For this review, take the finished solid that the model builds, in its own axes (mm). Face numbers are marked on the shaded views. A direction names the side the tool comes from. Coordinates: 2 decimals unless noted, no trailing zeros. Write each loop counter-clockwise with the first axis right and the second up, starting at its lowest first coordinate (ties: lowest second). Pieces come first, ordered by that corner, then holes. Notation, with made-up numbers: M 24,76 L 40,76 A27 ccw 40,108 Z; hole C 81,57 d7. An arc over 180 degrees is marked long. One line per question, with ' | ' between items.
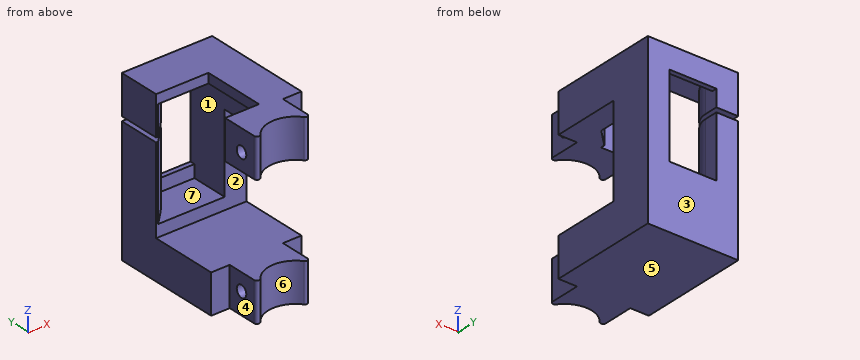
Autodesk Inventor part; units mm, degrees
ref_plane "YZ Plane" through (0, 0, 0) normal (1, 0, 0) x (0, 1, 0)
ref_plane "XZ Plane" through (0, 0, 0) normal (0, 1, 0) x (-1, 0, 0)
ref_plane "XY Plane" through (0, 0, 0) normal (0, 0, 1) x (1, 0, 0)
sketch "Side Block" plane through (0, 0, 0) normal (0, 0, 1) x (1, 0, 0)
  line L0 (11.2978, -7.5275) -> (11.2978, -16.0456)
  line L1 (11.2978, -7.5275) -> (16.5429, -7.5275)
  line L2 (16.5429, -7.5275) -> (16.5429, 23.5875)
  line L3 (16.5429, 23.5875) -> (-8.9841, 23.5875)
  line L4 (-8.9841, 23.5875) -> (-8.9841, -7.5275)
  line L5 (-8.9841, -7.5275) -> (-3.739, -7.5275)
  line L6 (-3.739, -16.0456) -> (-3.739, -7.5275)
  line L7 (3.7794, -23.2501) -> (3.7794, -21.2181)
  arc A0 (9.9308, -16.5088) -> (-2.3719, -16.5088) centre (3.7794, -21.2181) ccw
  arc A1 (-3.739, -16.0456) -> (-2.3719, -16.5088) centre (-2.977, -16.0456) ccw
  arc A2 (9.9308, -16.5088) -> (11.2978, -16.0456) centre (10.5358, -16.0456) ccw
  point P0 (3.7794, -4.0139)
  point P1 (-3.739, -19.35)
  point P2 (11.2978, -19.35)
  dimension "d2" = 31.115
  dimension "d3" = 31.115
  dimension "d4" = 5.2451
  dimension "d5" = 25.527
  dimension "d58" = 2.032
  dimension "d59" = 15.494
  dimension "d60" = 0.762
sketch "Motor Containment" plane through (0, 0, 0) normal (0, 0, 1) x (1, 0, 0)
  line L0 (-35.1538, -13.4444) -> (-35.1538, -17.0004) construction
  line L1 (-35.1538, -40.3684) -> (-35.1538, -43.9244) construction
  line L2 (-35.1538, -17.0004) -> (-35.1538, -22.8424)
  line L3 (-41.7578, -43.9244) -> (-28.5498, -43.9244)
  line L4 (-28.5498, -43.9244) -> (-28.5498, -13.4444)
  line L5 (-28.5498, -13.4444) -> (-41.7578, -13.4444)
  line L6 (-41.7578, -13.4444) -> (-41.7578, -43.9244)
  line L7 (-41.7578, -40.3684) -> (-28.5498, -40.3684)
  line L8 (-28.5498, -40.3684) -> (-28.5498, -17.0004)
  line L9 (-28.5498, -17.0004) -> (-41.7578, -17.0004)
  line L10 (-41.7578, -17.0004) -> (-41.7578, -40.3684)
  point P0 (-35.1538, -28.1145)
  dimension "d17" = 13.208
  dimension "d18" = 30.48
  dimension "d19" = 23.368
  dimension "d20" = 5.842
sketch "Sketch1" plane through (0, 0, 0) normal (0, 0, 1) x (1, 0, 0)
  line L0 (11.2978, -7.5275) -> (11.2978, -16.0456)
  line L1 (11.2978, -7.5275) -> (16.5429, -7.5275)
  line L2 (16.5429, -7.5275) -> (16.5429, 23.5875)
  line L3 (16.5429, 23.5875) -> (-8.9841, 23.5875)
  line L4 (-8.9841, 23.5875) -> (-8.9841, -7.5275)
  line L5 (-8.9841, -7.5275) -> (-3.739, -7.5275)
  line L6 (-3.739, -16.0456) -> (-3.739, -7.5275)
  line L7 (3.7794, -23.2501) -> (3.7794, -21.2181)
  arc A0 (9.9308, -16.5088) -> (-2.3719, -16.5088) centre (3.7794, -21.2181) ccw
  arc A1 (-3.739, -16.0456) -> (-2.3719, -16.5088) centre (-2.977, -16.0456) ccw
  arc A2 (9.9308, -16.5088) -> (11.2978, -16.0456) centre (10.5358, -16.0456) ccw
  point P0 (0, 0)
  dimension "d6" = 23.5875
extrude "Extrusion1" add sketch "Sketch1" along normal blind 47.5742
sketch "Sketch2" plane through (-8.9841, 23.5875, 0) normal (0, 1, 0) x (1, 0, 0)
  line L0 (0, -47.5742) -> (5.2451, -47.5742)
  line L1 (20.2819, 0) -> (25.527, 0)
  line L2 (0, -47.5742) -> (25.527, -47.5742)
  line L3 (25.527, -47.5742) -> (25.527, 0)
  line L4 (25.527, 0) -> (0, 0)
  line L5 (0, 0) -> (0, -47.5742)
  line L6 (0, -23.7871) -> (25.527, -23.7871) construction
  circle A0 centre (12.7635, -23.7871) radius 12.7
  line L7 (0, 0) -> (0, -47.5742)
  line L8 (0, -11.0871) -> (25.527, -11.0871)
  line L9 (12.7635, -14.3891) -> (12.7635, -17.9451) construction
  line L10 (12.7635, -41.3131) -> (12.7635, -44.8691) construction
  line L11 (12.7635, -17.9451) -> (12.7635, -23.7871)
  line L12 (6.1595, -44.8691) -> (19.3675, -44.8691)
  line L13 (19.3675, -44.8691) -> (19.3675, -14.3891)
  line L14 (19.3675, -14.3891) -> (6.1595, -14.3891)
  line L15 (6.1595, -14.3891) -> (6.1595, -44.8691)
  line L16 (6.1595, -41.3131) -> (19.3675, -41.3131)
  line L17 (19.3675, -41.3131) -> (19.3675, -17.9451)
  line L18 (19.3675, -17.9451) -> (6.1595, -17.9451)
  line L19 (6.1595, -17.9451) -> (6.1595, -41.3131)
  point P0 (8.9841, 0)
  point P1 (6.1595, -17.9451)
  dimension "d21" = 25.4
sketch "Sketch3" plane through (-8.9841, -7.5275, 0) normal (-1, 0, 0) x (0, 0, 1)
  line L0 (0, 19.177) -> (47.5742, 19.177)
  line L1 (47.5742, 31.115) -> (47.5742, 0)
  line L2 (0, 31.115) -> (47.5742, 31.115)
  line L3 (41.4528, 31.115) -> (41.4528, -19.3537) construction
  line L4 (6.1214, 31.115) -> (6.1214, -20.7554) construction
  line L5 (0, 31.115) -> (0, 0) construction
  circle A0 centre (6.1214, -4.1148) radius 1.6637
  circle A1 centre (41.4528, -4.1148) radius 1.6637
  line L6 (23.7871, 31.115) -> (23.7871, -19.3537) construction
  line L7 (36.576, 19.177) -> (36.576, -23.6144)
  line L8 (10.9982, 19.177) -> (10.9982, -23.6144)
  line L9 (36.576, -23.6144) -> (10.9982, -23.6144)
  line L10 (0, 0) -> (47.5742, 0)
  point P0 (10.9982, 19.177)
  dimension "d26" = 11.938
  dimension "d27" = 6.1214
  dimension "d28" = 6.1214
  dimension "d29" = 3.3274
  dimension "d30" = 3.3274
  dimension "d33" = 10.9982
  dimension "d54" = 4.1148
  dimension "d55" = 4.1148
extrude "Extrusion4" cut sketch "Sketch3" against normal blind 46.0375 contours L0 L7 L10 L8 | L10 L7 L9 L8 | A0 | A1
extrude "Extrusion5" cut sketch "Sketch2" against normal blind 23.8125 contours L15 L18 L13 A0 | A0 L13 L16 L15 | L15 L14 L13 L18 | L16 L13 L12 L15
sketch "Sketch4" plane through (0, 0, 47.5742) normal (0, 0, 1) x (1, 0, 0)
  line L0 (16.5429, 23.5875) -> (-8.9841, 23.5875) construction
  line L1 (3.7794, 23.5875) -> (3.7794, -25.467) construction
  line L2 (5.8114, 11.6495) -> (5.8114, -5.94)
  line L3 (-8.9841, 11.6495) -> (-8.9841, -7.5275)
  line L4 (-8.9841, -5.94) -> (16.5429, -5.94)
  line L5 (16.5429, -7.5275) -> (16.5429, 11.6495)
  line L6 (-8.9841, -7.5275) -> (-3.739, -7.5275)
  line L7 (-8.9841, 11.6495) -> (-2.8246, 11.6495)
  line L8 (-8.9841, 11.6495) -> (5.8114, 11.6495)
  line L9 (-3.739, -7.5275) -> (-3.739, -16.0456)
  line L10 (-3.739, -7.5275) -> (-3.739, -5.94)
  point P0 (0, 0)
  point P1 (-3.739, -18.0776)
  dimension "d38" = 2.032
  dimension "d39" = 1.5875
extrude "Extrusion6" cut sketch "Sketch4" against normal blind 14.2875
chamfer "Chamfer1" distance 5.588 angle 45 1 edges at (-2.8246, 11.6495, 29.6291)
sketch "Sketch5" plane through (3.7794, -23.2501, 36.576) normal (0, 0, -1) x (-1, 0, 0)
  line L0 (-6.604, 23.0251) -> (-6.604, 34.8996)
  line L1 (-6.604, 23.0251) -> (-2.032, 18.4531)
  line L2 (-2.032, 17.3101) -> (-2.032, 23.0251)
  line L3 (-6.604, 23.0251) -> (-0.1382, 23.0251) construction
  line L4 (-2.032, 18.4531) -> (-2.032, 23.0251)
  line L5 (-2.032, 23.0251) -> (-6.604, 23.0251)
  point P0 (3.7794, 23.2501)
  dimension "d45" = 45
extrude "Extrusion7" cut sketch "Sketch5" against normal up to surface (8.2931 mm away)
extrude "Extrusion8" add sketch "Sketch2" against normal blind 1.397 contours L15 L14 L13 L18 | L16 L13 L12 L15
sketch "Sketch6" plane through (-8.9841, -7.5275, 0) normal (-1, 0, 0) x (0, 0, 1)
  line L0 (0, 31.115) -> (47.5742, 31.115)
  line L1 (36.576, 19.177) -> (14.3891, 19.177)
  line L2 (36.576, 31.115) -> (35.306, 31.115)
  line L3 (35.306, 31.115) -> (35.306, 19.177)
  line L4 (35.306, 19.177) -> (36.576, 19.177)
  line L5 (36.576, 19.177) -> (36.576, 31.115)
  line L6 (36.576, 7.3025) -> (36.576, 19.177)
  point P0 (0, 7.5275)
  dimension "d52" = 0
  dimension "d53" = 1.27
extrude "Extrusion9" cut sketch "Sketch6" against normal blind 14.2875
fillet "Fillet1" radius 6.35 2 edges at (-2.8246, 17.2375, 40.7226) (-2.8246, 17.2375, 24.8476)
equation "\"d27\" = d28"
equation "\"d30\" = d29"
properties part number "Servo Mount V5"
1. Clearance check with flat-ended pins moving along their axes: P1, Ø12, axis at y = 3.5, z = 43, coming from the -X side; P2, Ø8, axis at y = -10, z = 42, coming from the -X side; P3, Ø10, axis at x = 5, z = 24, coming from the -Y side; P4, Ø4.5, axis at y = -12, z = 39.5, coming from the +X side. State where each tip first meets the part, or that it passes through.
Computed values:
P1: stops at x = 5.81 | P2: stops at x = -3.74 | P3: passes through | P4: stops at x = 11.3
2. For line 1 along Z through (x, y) = (-7, 12.5); line 2 along Z through (x, y) = (9, -10.5); line 3 along Z through (x, y) = (9.75, -9.5), list the stretches that pass through material, from the lowest coordinate up.
Computed values:
line 1: z = 0 to 14.39, 44.87 to 47.57 | line 2: z = 0 to 4.91, 7.33 to 11, 36.58 to 40.24, 42.66 to 47.57 | line 3: z = 0 to 11, 36.58 to 47.57
3. Take a section at C-C on x = -1.25. State the section outline as (y, z) points.
Computed values:
outline: M -15.33,0 L 23.59,0 L 23.59,17.95 L 22.19,17.95 L 22.19,14.39 L 11.65,14.39 L 11.65,11 L -15.33,11 Z; M -15.33,36.58 L -5.94,36.58 L -5.94,47.57 L -15.33,47.57 Z; M 11.65,44.87 L 22.19,44.87 L 22.19,41.31 L 23.59,41.31 L 23.59,47.57 L 11.65,47.57 Z; hole C -11.64,6.12 d3.33; hole C -11.64,41.45 d3.33
4. Draft analysis for pull direction Z (two halves, no side actions). For the marked faces 5, 6 and 7, state which applies: pulls with the +Z half, pulls with the -Z half, needs draft (parallel to the pull), parting line crosses it, or undercut.
Computed values:
face 5: pulls with the -Z half | face 6: needs draft | face 7: undercut
5. Take a section at A-A on z = 31. State the section outline as (x, y) points, plus the area to 3 significant figures.
Computed values:
outline: M -8.98,11.65 L -8.41,11.65 L -4.68,15.38 A6.35 ccw -2.82,19.87 L -2.82,23.59 L -8.98,23.59 Z; M 10.38,11.65 L 16.54,11.65 L 16.54,23.59 L 10.38,23.59 Z | area: 131 mm2
6. Take a section at B-B on y = 10. State the section outline as (x, z) points.
Computed values:
outline: M -8.98,0 L 16.54,0 L 16.54,11 L -8.98,11 Z; M 5.81,44.87 L 10.38,44.87 L 10.38,36.58 L 16.54,36.58 L 16.54,47.57 L 5.81,47.57 Z
7. Machinability: for the marked faces 1, 2, 3 and 4, which of the approach directions +Z, -Z, +X, -X, +Y, -Y give a long, thin tool a straight path to every point of the face, cutting with its end or side? Answer none if there is none.
Computed values:
face 1: none | face 2: +X, -X, -Y | face 3: +Z, -Z, +X, -X, +Y | face 4: +Z, -Z, -X, -Y
8. Take a section at D-D on z = 8.5. State the section outline as (x, y) points.
Computed values:
outline: M -8.98,-7.53 L -3.74,-7.53 L -3.74,-16.05 A0.76 ccw -2.37,-16.51 A7.75 cw 9.93,-16.51 A0.76 ccw 11.3,-16.05 L 11.3,-7.53 L 16.54,-7.53 L 16.54,23.59 L -8.98,23.59 Z
